Answer from the drawing. Dimensions are ordinates in mm from the lowest x, y and z of the part. Coordinates: 2 decimals unless noted, no trailing zeros. Order: outer loops, then holes, each group sorted by start corner. A loop starts at its lowest first (then second) coordinate and runs counter-clockwise, first axis right, second up. Notation, with made-up numbers: (34, -22) - (59, -22) arc R26 ccw to (59, 3) - close; hole circle Ø6 at (-3.75, 54). An arc over 180 degrees is marked (long way). One line per item, written item: value. Start each with the question number.
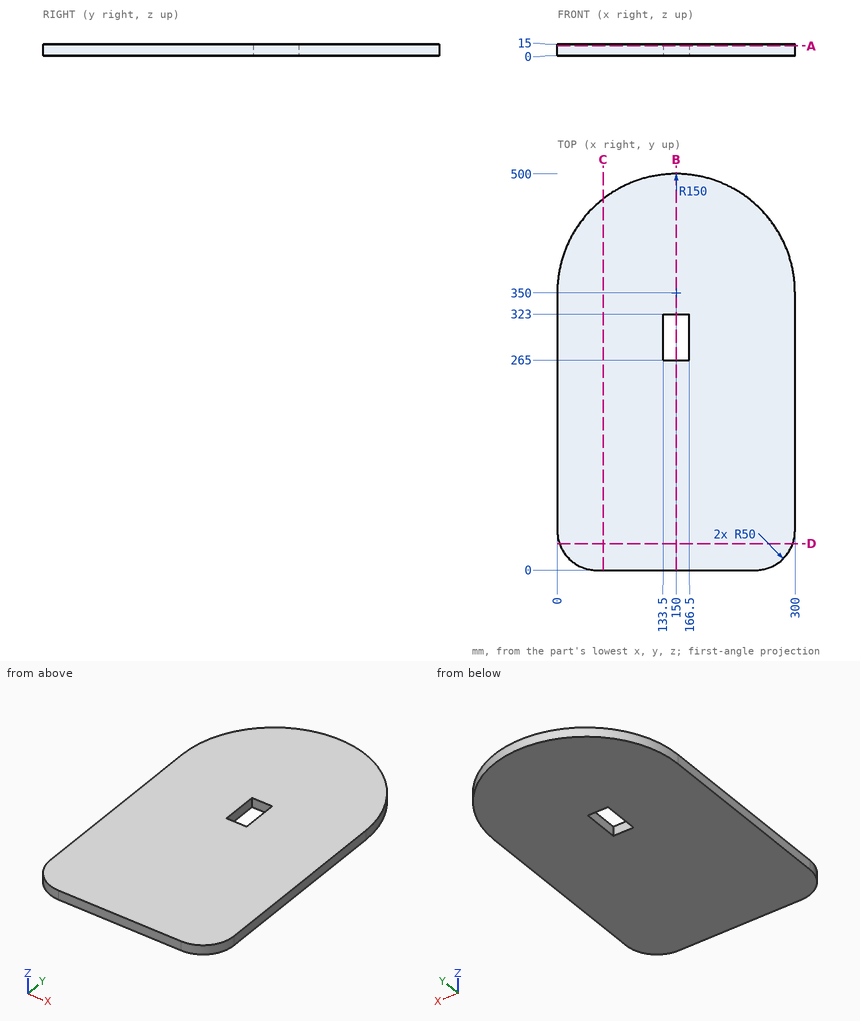
(1) The part is cut by section D-D on y = 33.5. Determine the outline of the cut face in (x, z), plus the area to 3 significant figures.
(2) The part is cut by section B-B on x = 150. Determine the outline of the cut face in (y, z), plus the area to 3 significant figures.
(3) Consider probe 1 along Y at (x, z) = (134, 1); probe 2 along X at (y, z) = (266, 7.5); probe 3 along X at (y, z) = (439, 9.5). Determine where each line is inside the solid, lowest interval first.
(4) The part is cut by section C-C on x = 58. Determine the outline of the cut face in (y, z), plus the area to 3 significant figures.
(5) Flat-ended cylindrical pins translate along their axes: pin 1 Ø7.5 at (x, z) = (144.5, 8) entering from +Y; pin 2 Ø5 at (x, z) = (50.5, 13) entering from +Y; pin 3 Ø5 at (y, z) = (437.5, 12.5) entering from -X. Find the tip coordinate at first contact, or state that the pin passes through.
(6) The part is cut by section A-A on z = 12.5. Determine the outline of the cut face in (x, y), plus the area to 3 significant figures.
Completed:
1. outline: (2.8, 0) - (297.2, 0) - (297.2, 15) - (2.8, 15) - close
1. area: 4,420 mm2
2. outline: (0, 0) - (265, 0) - (265, 15) - (0, 15) - close; (323, 0) - (500, 0) - (500, 15) - (323, 15) - close
2. area: 6,630 mm2
3. probe 1: y = 0 to 265, 323 to 499.14
3. probe 2: x = 0 to 133.5, 166.5 to 300
3. probe 3: x = 29.26 to 270.74
4. outline: (0, 0) - (468.47, 0) - (468.47, 15) - (0, 15) - close
4. area: 7,030 mm2
5. pin 1: stops at y = 499.99
5. pin 2: stops at y = 464.42
5. pin 3: stops at x = 26.41
6. outline: (0, 50) arc R50 ccw to (50, 0) - (250, 0) arc R50 ccw to (300, 50) - (300, 350) arc R150 ccw to (0, 350) - close; hole (133.5, 265) - (166.5, 265) - (166.5, 323) - (133.5, 323) - close
6. area: 137,000 mm2
